Source: CAD feature listing. Evaluate the final solid. Frame: model axes, mm. Coordinates: 2 decimals unless noted, no trailing zeros. Loops run counter-clockwise (first coordinate to the right, second up) from the corner with the lowest first, then second, coordinate; pieces in that order, holes last. Notation, with made-up numbers: (1, 28.25) - (12, 28.25) arc R11 ccw to (12, 45.25) - close; hole circle Ø11 at (-8, 25.25). An arc over 180 degrees is marked (long way). Use one line per item in the form item = value. Start each with the question number.
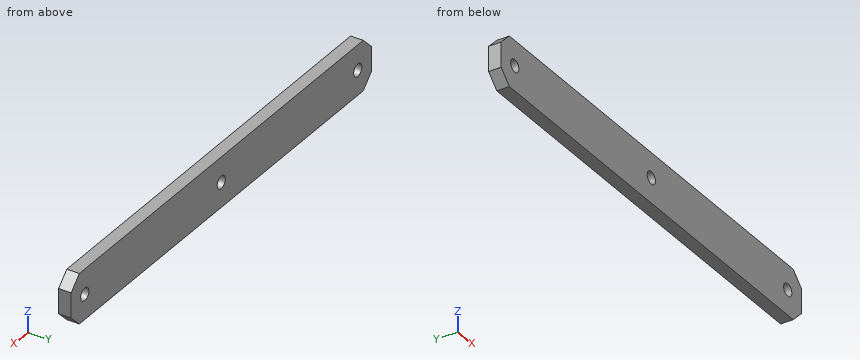
from build123d import *

# Parameters (mm, degrees)
SKETCH1_R           = 1.5
BOSS_EXTRUDE1_DEPTH = 3


with BuildPart() as part:
    # Sketch1 → Boss-Extrude1 (new body)
    with BuildSketch(Plane(origin=(0, 0, 0), x_dir=(1, 0, 0), z_dir=(0, 1, 0))):
        Polygon((-55, 3), (-52, 6), (52, 6), (55, 3), (55, -3), (52, -6), (-52, -6), (-55, -3), align=None)
        with Locations(Location((-50, 0, 0), (0, 0, 270))):
            Circle(SKETCH1_R, mode=Mode.SUBTRACT)
        with Locations(Location((0, 0, 0), (0, 0, 270))):
            Circle(SKETCH1_R, mode=Mode.SUBTRACT)
        with Locations(Location((50, 0, 0), (0, 0, 270))):
            Circle(SKETCH1_R, mode=Mode.SUBTRACT)
    extrude(amount=BOSS_EXTRUDE1_DEPTH)


solid = part.part
(1) Cut plane C-C, the plane z = 0. Output: boundary loops of the cut face in (x, y).
(2) Contact query for a flat-ended pin moving along its axis: pin 1 (1.8 mm diameter, centred on x = 0, z = 0, fed in from -Y). Output: stop coordinate, or through.
(3) Cut plane B-B, the plane y = 0.9. Output: boundary loops of the cut face in (x, z), plus the area to 3 significant figures.
(4) Material intervals for line 1 (X direction, y = 1.75, z = 0); line 2 (X direction, y = 1.95, z = -1); line 3 (X direction, y = 2.8, z = -4.25), sorted ascending.
(5) Cut plane A-A, the plane x = 50. Output: boundary loops of the cut face in (y, z).
Recorded:
q1.outline = (-55, 0) - (-51.5, 0) - (-51.5, 3) - (-55, 3) - close; (-48.5, 0) - (-1.5, 0) - (-1.5, 3) - (-48.5, 3) - close; (1.5, 0) - (48.5, 0) - (48.5, 3) - (1.5, 3) - close; (51.5, 0) - (55, 0) - (55, 3) - (51.5, 3) - close
q2.pin_1 = through
q3.outline = (-55, -3) - (-52, -6) - (52, -6) - (55, -3) - (55, 3) - (52, 6) - (-52, 6) - (-55, 3) - close; hole circle Ø3 at (-50, 0); hole circle Ø3 at (0, 0); hole circle Ø3 at (50, 0)
q3.area = 1,280 mm²
q4.line_1 = -55 to -51.5, -48.5 to -1.5, 1.5 to 48.5, 51.5 to 55
q4.line_2 = -55 to -51.12, -48.88 to -1.12, 1.12 to 48.88, 51.12 to 55
q4.line_3 = -53.75 to 53.75
q5.outline = (0, -6) - (3, -6) - (3, -1.5) - (0, -1.5) - close; (0, 1.5) - (3, 1.5) - (3, 6) - (0, 6) - close
